Geometry: final body of the model. Coordinates: model frame, mm. A direction names the side the tool comes from. Coordinates: 2 decimals unless noted, no trailing zeros. Write each loop counter-clockwise with the first axis right and the second up, starting at its lowest first coordinate (ties: lowest second). Pieces come first, ordered by that corner, then holes.
Autodesk Inventor part; units mm, degrees
ref_plane "YZ Plane" through (0, 0, 0) normal (1, 0, 0) x (0, 1, 0)
ref_plane "XZ Plane" through (0, 0, 0) normal (0, 1, 0) x (-1, 0, 0)
ref_plane "XY Plane" through (0, 0, 0) normal (0, 0, 1) x (1, 0, 0)
sketch "Sketch1" plane through (0, 0, 0) normal (0, 0, 1) x (1, 0, 0)
  line L0 (0, 0) -> (55, 0)
  line L1 (55, 0) -> (55, 50)
  line L2 (55, 50) -> (0, 50)
  line L3 (0, 50) -> (0, 0)
  dimension "d0" = 55
  dimension "d1" = 50
extrude "Extrusion1" add sketch "Sketch1" along normal blind 5
sketch "Sketch2" plane through (0, 0, 5) normal (0, 0, 1) x (1, 0, 0)
  line L0 (55, 0) -> (0, 0)
  line L1 (55, 50) -> (55, 0)
  line L2 (20, 15) -> (50, 15)
  line L3 (50, 15) -> (50, 35)
  line L4 (50, 35) -> (20, 35)
  line L5 (20, 35) -> (20, 15)
  dimension "d4" = 30
  dimension "d5" = 20
  dimension "d6" = 5
  dimension "d7" = 15
extrude "Extrusion2" cut sketch "Sketch2" against normal blind 5
sketch "Sketch3" plane through (0, 0, 5) normal (0, 0, 1) x (1, 0, 0)
  circle A0 centre (20, 35) radius 1
  circle A1 centre (20, 15) radius 1
  circle A2 centre (50, 15) radius 1
  circle A3 centre (50, 35) radius 1
  point P0 (50, 35)
  point P1 (20, 15)
  dimension "d10" = 2
  dimension "d11" = 2
  dimension "d12" = 2
  dimension "d13" = 2
hole "Hole1" at (20, 35, 5) at (20, 15, 5) at (50, 15, 5) at (50, 35, 5) direction (0, 0, -1) diameter 2 depth 5 tip angle 118
sketch "Sketch4" plane through (0, 0, 5) normal (0, 0, 1) x (1, 0, 0)
  line L0 (0, 0) -> (0, 50)
  line L1 (55, 0) -> (0, 0)
  line L2 (55, 50) -> (55, 0)
  line L3 (0, 50) -> (55, 50)
  point P0 (8, 25)
  point P1 (47, 42.5)
  point P2 (47, 7.5)
  dimension "d21" = 35
  dimension "d22" = 7.5
  dimension "d23" = 8
  dimension "d24" = 8
  dimension "d25" = 8
  dimension "d26" = 25
hole "Hole2" at (8, 25, 5) at (47, 42.5, 5) at (47, 7.5, 5) direction (0, 0, -1) diameter 6.5 depth 5 tip angle 118 countersink diameter 11.5 countersink angle 90
properties part number "ASSOALHO(8)" material "Carbon Steel"
Item 1: Material intervals for probe 1 along X at (y, z) = (25, 0.9); probe 2 along X at (y, z) = (7.5, 2); probe 3 along Y at (x, z) = (47.5, 0.85), sorted ascending.
Derived:
probe 1: x = 0 to 4.75, 11.25 to 20, 50 to 55
probe 2: x = 0 to 43.75, 50.25 to 55
probe 3: y = 0 to 4.29, 10.71 to 15, 35 to 39.29, 45.71 to 50
Item 2: Set-up query: faces 4 (the conical face through (43.978, 5.928, 2.656)), 5 (the flat face through (35, 15, 3)). Return all of +Z, -Z, +X, -X, +Y, -Y with unobstructed straight access to the full face (end or side cutting, diameter ignored); none if empty.
Derived:
face 4: +Z
face 5: +Z, -Z
Item 3: Section B-B, the plane z = 3.9. Output: boundary loops of the cut face in (x, y), plus the area to 3 significant figures.
Derived:
outline: (0, 0) - (55, 0) - (55, 50) - (0, 50) - close; hole circle Ø9.3 at (8, 25); hole (20, 16) arc R1 ccw (long way) to (21, 15) - (49, 15) arc R1 ccw (long way) to (50, 16) - (50, 34) arc R1 ccw (long way) to (49, 35) - (21, 35) arc R1 ccw (long way) to (20, 34) - close; hole circle Ø9.3 at (47, 7.5); hole circle Ø9.3 at (47, 42.5)
area: 1,940 mm2
Item 4: Section C-C, the plane y = 7.5. Output: boundary loops of the cut face in (x, z), plus the area to 3 significant figures.
Derived:
outline: (0, 0) - (43.75, 0) - (43.75, 2.5) - (41.25, 5) - (0, 5) - close; (50.25, 0) - (55, 0) - (55, 5) - (52.75, 5) - (50.25, 2.5) - close
area: 236 mm2
Item 5: Section A-A, the plane y = 25. Output: boundary loops of the cut face in (x, z).
Derived:
outline: (0, 0) - (4.75, 0) - (4.75, 2.5) - (2.25, 5) - (0, 5) - close; (11.25, 0) - (20, 0) - (20, 5) - (13.75, 5) - (11.25, 2.5) - close; (50, 0) - (55, 0) - (55, 5) - (50, 5) - close
Item 6: Pull-direction query (X, two-part tool) for faces 1 (the flat face through (28, 50, 2)), 2 (the flat face through (50, 25, 3)), 3 (the flat face through (0, 25, 2)); classes: released by +X, released by -X, zero draft, split by the parting line, or undercut.
Derived:
face 1: zero draft
face 2: undercut
face 3: released by -X
Item 7: Section D-D, the plane x = 36. Output: boundary loops of the cut face in (y, z), plus the area to 3 significant figures.
Derived:
outline: (0, 0) - (15, 0) - (15, 5) - (0, 5) - close; (35, 0) - (50, 0) - (50, 5) - (35, 5) - close
area: 150 mm2
Item 8: Pin query (flat end, axial travel): pin 1 (4 mm diameter, centred on x = 47, y = 42.5, fed in from +Z); pin 2 (8 mm diameter, centred on x = 45, y = 32, fed in from +Z); pin 3 (8.5 mm diameter, centred on x = 8, y = 25, fed in from +Z). Return the tip coordinate at first contact, or that it passes through.
Derived:
pin 1: passes through
pin 2: stops at z = 5
pin 3: stops at z = 3.5
